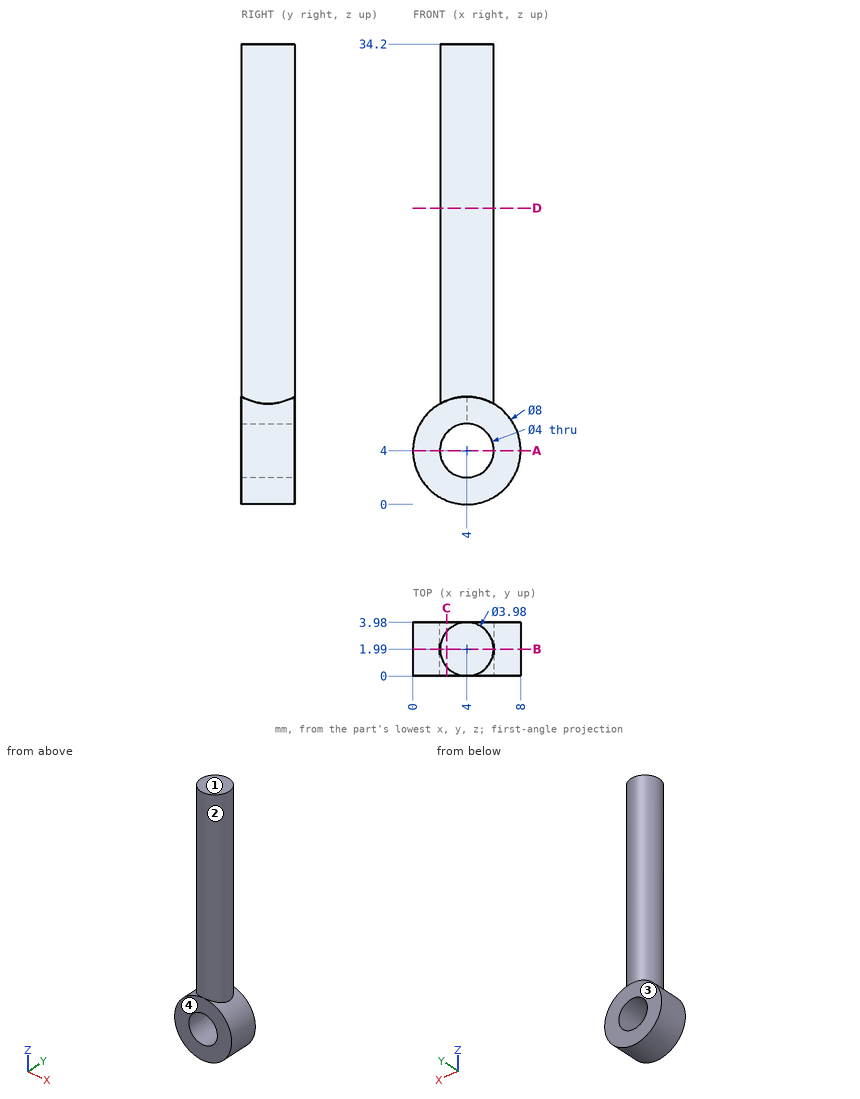
Answer from the drawing. Dimensions are ordinates in mm from the lowest x, y and z of the part. Round coordinates to 2 decimals unless told otherwise and drop trailing zeros. Loops run counter-clockwise (first coordinate to the right, second up) from the corner with the lowest first, then second, coordinate; pieces in that order, holes last.
Q1. Section A-A on z = 4 is taken. Write down the section's boundary in (x, y), and give its area (3 significant figures).
Q2. Section C-C on x = 2.5 is taken. Write down the section's boundary in (y, z), and give its area (3 significant figures).
Q3. Section D-D on z = 22 is taken. Write down the section's boundary in (x, y).
Q4. Each of these flat-tipped pins is pushed along its axis until it touches: pin 1 (1 mm diameter, centred on x = 5, y = 2, fed in from -Z); pin 2 (1.5 mm diameter, centred on x = 6, y = 2.5, fed in from -Z); pin 3 (4 mm diameter, centred on x = 2.5, z = 10, fed in from +Y). Where does it stop, or does it pass through?
Q5. Section B-B on y = 1.99 is taken. Write down the section's boundary in (x, z).
Q6. Consider probe 1 along Z at (x, y) = (4, 1.15); probe 2 along X at (y, z) = (3.45, 2.5); probe 3 along Z at (x, y) = (4.75, 3.2). Determine where each line is inside the solid, lowest interval first.
Q7. Determine the mould class of the marked faces 1, 2, 3 and 4 for opening direction Y: released by +Y, released by -Y, zero draft, split by the parting line, or undercut.
Output:
1. outline: (0, 0) - (2, 0) - (2, 3.98) - (0, 3.98) - close; (6, 0) - (8, 0) - (8, 3.98) - (6, 3.98) - close
1. area: 15.9 mm2
2. outline: (0, 0.29) - (3.98, 0.29) - (3.98, 2.68) - (0, 2.68) - close; (0, 5.32) - (3.98, 5.32) - (3.98, 7.71) - (3.3, 7.71) - (3.3, 34.2) - (0.68, 34.2) - (0.68, 7.71) - (0, 7.71) - close
2. area: 88.3 mm2
3. outline: circle Ø3.98 at (4, 1.99)
4. pin 1: stops at z = 0.03
4. pin 2: stops at z = 0.2
4. pin 3: stops at y = 3.98
5. outline: (2.01, 7.47) arc R4 ccw (long way) to (5.99, 7.47) - (5.99, 34.2) - (2.01, 34.2) - close; hole circle Ø4 at (4, 4)
6. probe 1: z = 0 to 2, 6 to 34.2
6. probe 2: x = 0.29 to 2.68, 5.32 to 7.71
6. probe 3: z = 0.07 to 2.15, 5.85 to 34.2
7. face 1: zero draft
7. face 2: split by the parting line
7. face 3: released by +Y
7. face 4: released by -Y
